Read the model definition and answer for the solid it produces. Units are mm, in the model's axes. Face numbers are marked on the shaded views. A direction names the side the tool comes from. Give positions to 0.01 mm unless a question says otherwise; leave off trailing zeros. Order: outer loops, then holes, each group sorted by start corner. A loop starts at its lowest first (then second) coordinate and runs counter-clockwise, first axis right, second up.
Item 1: A cutting plane is placed at D-D (x = 8). Write down the section's boundary in (y, z) (3 decimals), plus the area to 3 significant figures.
Item 2: A cutting plane is placed at C-C (x = 3.5). Write down the section's boundary in (y, z) (3 decimals).
Item 3: A cutting plane is placed at B-B (z = -2). Write down the section's boundary in (x, y) (3 decimals).
Item 4: Given pin 1 Ø2 at (x, z) = (7.5, -8) entering from +Y, flat-ended and moving along its own axis, determine where the tip first touches the part or whether it passes through.
Item 5: Find the intervals of material crossed by line 1 along X through (y, z) = (0.8, -1.5) (3 decimals); line 2 along Z through (x, y) = (6.5, 0.45) (3 decimals); line 3 along Z through (x, y) = (10.25, 0.7) (3 decimals), in increasing order.
Item 6: A cutting plane is placed at A-A (y = 1.1). Write down the section's boundary in (x, z) (3 decimals), plus the area to 3 significant figures.
Item 7: The mould has two halves that part along Z. Classify the marked faces 3, 4 and 5: +Z half, -Z half, draft (parallel to the pull), parting line (faces both ways), or undercut.
Item 8: Which of the six approach directions +Z, -Z, +X, -X, +Y, -Y give full straight-line access (tool end or side, diameter ignored) to the marked faces 1 and 2?
from build123d import *

# Parameters (mm, degrees)
SKETCH1_W           = 12.7
SKETCH1_H           = 12.7
BOSS_EXTRUDE1_DEPTH = 2.54
FILLET1_R           = 0.635
SHELL1_START        = 0.635
SHELL1_OUTLINE_W    = 1.905
SHELL1_OUTLINE_H    = 11.43
SHELL1_DEPTH        = 11.43
SKETCH2_R           = 2.54
BOSS_EXTRUDE2_DEPTH = 1.905
BOSS_EXTRUDE3_DEPTH = 0.00254


# Read off the part's stored shape, not the designer's step: Shell1
with BuildPart() as part:
    # Sketch1 → Boss-Extrude1 (new body)
    with BuildSketch(Plane(origin=(0, 0, 0), x_dir=(1, 0, 0), z_dir=(0, 1, 0))):
        with Locations((6.35, 6.35)):
            Rectangle(SKETCH1_W, SKETCH1_H)
    extrude(amount=BOSS_EXTRUDE1_DEPTH)

    # Fillet1
    fillet1_edges = [part.edges().sort_by_distance(p)[0] for p in [
        (0, 1.27, -12.7),
        (12.7, 1.27, -12.7),
        (12.7, 1.27, 0),
        (0, 1.27, 0),
    ]]
    fillet(fillet1_edges, radius=FILLET1_R)

    # Shell1 outline → Shell1 (cut)
    with BuildSketch(Plane.YZ.offset(SHELL1_START)):
        with Locations((0.9525, -6.35)):
            Rectangle(SHELL1_OUTLINE_W, SHELL1_OUTLINE_H)
    extrude(amount=SHELL1_DEPTH, mode=Mode.SUBTRACT)

    # Sketch2 → Boss-Extrude2 (add)
    with BuildSketch(Plane(origin=(0, 1.905, 0), x_dir=(-1, 0, 0), z_dir=(0, -1, 0))):
        with Locations(Location((-6.35, 6.35, 0), (0, 0, 270))):
            Circle(SKETCH2_R)
    extrude(amount=BOSS_EXTRUDE2_DEPTH)

    # Sketch3 → Boss-Extrude3 (add)
    with BuildSketch(Plane(origin=(0, 2.54, 0), x_dir=(1, 0, 0), z_dir=(0, 1, 0))):
        with BuildLine():
            Line((6.947551282, 7.576776242), (6.521419471, 7.186897436))
            add(Edge.make_bspline(
                [(6.521419471, 7.186897436), (6.503165812, 7.21264612), (6.468121331, 7.262080004), (6.411317883, 7.328273139), (6.354770931, 7.384740809), (6.297956603, 7.431247119), (6.240371318, 7.467509507), (6.182115036, 7.493183679), (6.123518028, 7.509504993), (6.084149883, 7.51153739), (6.064758814, 7.512538462)],
                knots=[0, 0, 0, 0, 1.299362458, 2.494594718, 3.587462134, 4.587049575, 5.512617175, 6.380583204, 7.202344345, 8, 8, 8, 8], degree=3))
            add(Edge.make_bspline(
                [(6.064758814, 7.512538462), (6.046671381, 7.511904137), (6.0117493, 7.510679422), (5.961965283, 7.498505847), (5.917766323, 7.477496044), (5.879195557, 7.45002396), (5.84864182, 7.416926467), (5.82424703, 7.382215707), (5.810510714, 7.343902879), (5.808702744, 7.317588082), (5.807807692, 7.304560697)],
                knots=[0, 0, 0, 0, 1.185010067, 2.2879431, 3.333075148, 4.379039566, 5.372662701, 6.27520591, 7.14612461, 8, 8, 8, 8], degree=3))
            add(Edge.make_bspline(
                [(5.807807692, 7.304560697), (5.808368576, 7.291345451), (5.809498118, 7.264731783), (5.820407957, 7.225726137), (5.836852199, 7.18761308), (5.852565344, 7.164411849), (5.860597155, 7.152552484)],
                knots=[0, 0, 0, 0, 0.967525499, 1.948461899, 2.951351359, 4, 4, 4, 4], degree=3))
            add(Edge.make_bspline(
                [(5.860597155, 7.152552484), (5.867898941, 7.143334324), (5.884706688, 7.122115336), (5.916755618, 7.088507766), (5.957002343, 7.047335552), (6.006995642, 7.000014485), (6.064660156, 6.944842714), (6.132668709, 6.883989063), (6.209063719, 6.815568965), (6.263363522, 6.767923686), (6.291817107, 6.742957131)],
                knots=[0, 0, 0, 0, 0.473873513, 1.090794244, 1.870441696, 2.795289791, 3.865433203, 5.087734844, 6.473946851, 8, 8, 8, 8], degree=3))
            add(Edge.make_bspline(
                [(6.291817107, 6.742957131), (6.31852489, 6.719842892), (6.369210714, 6.675976869), (6.441326575, 6.613716092), (6.504704406, 6.557701589), (6.560267478, 6.508774018), (6.607173508, 6.466420016), (6.645619689, 6.430437133), (6.676075577, 6.401525888), (6.693387966, 6.384063478), (6.700776442, 6.376610978)],
                knots=[0, 0, 0, 0, 1.543621617, 2.929473131, 4.163658386, 5.240097082, 6.164993805, 6.925417477, 7.541396219, 8, 8, 8, 8], degree=3))
            add(Edge.make_bspline(
                [(6.700776442, 6.376610978), (6.72880678, 6.346276149), (6.782690932, 6.287961956), (6.852721334, 6.197593297), (6.910358621, 6.109375058), (6.954947919, 6.021647272), (6.98862355, 5.9331442), (7.012365316, 5.84169531), (7.026584417, 5.746345018), (7.02816307, 5.681280084), (7.028961538, 5.648370793)],
                knots=[0, 0, 0, 0, 1.206664779, 2.319633467, 3.337109185, 4.282041471, 5.190008762, 6.099243693, 7.03861361, 8, 8, 8, 8], degree=3))
            add(Edge.make_bspline(
                [(7.028961538, 5.648370793), (7.028393209, 5.616304725), (7.027278125, 5.553389906), (7.013620483, 5.46132344), (6.994145488, 5.373211837), (6.96403373, 5.290013874), (6.927333696, 5.210363884), (6.881324904, 5.135502559), (6.827293886, 5.064672272), (6.765366044, 4.999139201), (6.696866497, 4.939672482), (6.623394222, 4.886733804), (6.544230772, 4.843026182), (6.460052505, 4.807036073), (6.370904481, 4.77931601), (6.276892901, 4.7588283), (6.17787397, 4.746531899), (6.110163397, 4.745246456), (6.075571114, 4.744589744)],
                knots=[0, 0, 0, 0, 1.043214005, 2.046824704, 3.02475056, 3.976699089, 4.921714032, 5.875962561, 6.831408892, 7.817874052, 8.806269674, 9.781291748, 10.760897367, 11.74438705, 12.757449933, 13.795994037, 14.874007457, 16, 16, 16, 16], degree=3))
            add(Edge.make_bspline(
                [(6.075571114, 4.744589744), (6.048416466, 4.745071485), (5.994634689, 4.74602561), (5.915368481, 4.753815242), (5.838827997, 4.766386881), (5.765099453, 4.784405794), (5.693850688, 4.807238201), (5.625078777, 4.835127112), (5.559258474, 4.868504794), (5.495891752, 4.906684869), (5.435286652, 4.951016965), (5.376676846, 5.000594728), (5.320644503, 5.056180684), (5.266920509, 5.117643377), (5.215848607, 5.185156853), (5.165757029, 5.257780861), (5.118871997, 5.336863206), (5.089909027, 5.392340111), (5.075115385, 5.420676482)],
                knots=[0, 0, 0, 0, 1.016823716, 2.013894106, 2.979844003, 3.91962641, 4.853723003, 5.779685073, 6.695824784, 7.614987388, 8.547259901, 9.504950863, 10.487499108, 11.500346958, 12.559593716, 13.656357062, 14.802919212, 16, 16, 16, 16], degree=3))
            Line((5.075115385, 5.420676482), (5.576297276, 5.721512821))
            add(Edge.make_bspline(
                [(5.576297276, 5.721512821), (5.594801911, 5.689347337), (5.630276879, 5.627683355), (5.690392527, 5.54482998), (5.751977941, 5.473879779), (5.816456918, 5.416086802), (5.883045419, 5.370678281), (5.952065082, 5.338226202), (6.023564398, 5.318138402), (6.072266484, 5.315685218), (6.096559696, 5.314461538)],
                knots=[0, 0, 0, 0, 1.283663364, 2.460892379, 3.537111102, 4.529833553, 5.449777664, 6.316464042, 7.160231139, 8, 8, 8, 8], degree=3))
            add(Edge.make_bspline(
                [(6.096559696, 5.314461538), (6.12126937, 5.315460861), (6.169209736, 5.317399693), (6.237638475, 5.335308096), (6.300376534, 5.363425604), (6.354606849, 5.403545409), (6.40052566, 5.449849762), (6.434416378, 5.501365473), (6.455706756, 5.557104227), (6.457957665, 5.595824033), (6.459089744, 5.615297877)],
                knots=[0, 0, 0, 0, 1.13588714, 2.203786484, 3.234766741, 4.283437687, 5.291419208, 6.222934724, 7.106237994, 8, 8, 8, 8], degree=3))
            add(Edge.make_bspline(
                [(6.459089744, 5.615297877), (6.458044316, 5.633415119), (6.455920629, 5.670218563), (6.440278206, 5.724939365), (6.415824328, 5.779635282), (6.386893665, 5.824498352), (6.357453094, 5.862060985), (6.329301267, 5.894607307), (6.295019789, 5.930565296), (6.254695583, 5.969980182), (6.208861436, 6.013198947), (6.157478739, 6.060217356), (6.099959106, 6.110621236), (6.059304117, 6.14495586), (6.038046074, 6.162909054)],
                knots=[0, 0, 0, 0, 0.916159276, 1.861089862, 2.860218735, 3.940849679, 4.552606315, 5.27541173, 6.11797699, 7.06649574, 8.129236253, 9.306560635, 10.591630461, 12, 12, 12, 12], degree=3))
            add(Edge.make_bspline(
                [(6.038046074, 6.162909054), (5.997633688, 6.197101808), (5.920070088, 6.262728051), (5.810462881, 6.359655946), (5.711696974, 6.450243946), (5.624625414, 6.535611915), (5.548138776, 6.614183306), (5.482755059, 6.686596305), (5.429192535, 6.75340948), (5.372829528, 6.832545214), (5.319273403, 6.928977544), (5.272985712, 7.044996816), (5.242956212, 7.161001367), (5.239591824, 7.238880433), (5.237935897, 7.277211939)],
                knots=[0, 0, 0, 0, 1.345494975, 2.582412109, 3.71882943, 4.751509156, 5.681369928, 6.505683931, 7.230279997, 7.856715994, 8.973648664, 10.023341002, 11.027102913, 12, 12, 12, 12], degree=3))
            add(Edge.make_bspline(
                [(5.237935897, 7.277211939), (5.238624595, 7.304394586), (5.239981404, 7.35794732), (5.252084347, 7.436688812), (5.270172657, 7.512667736), (5.296442076, 7.585606886), (5.33053661, 7.655414903), (5.371943098, 7.722433526), (5.421304502, 7.786045931), (5.476931473, 7.846209948), (5.538218153, 7.901193012), (5.603710758, 7.949721076), (5.673038596, 7.990708584), (5.745777553, 8.024710699), (5.822378363, 8.050737157), (5.90227671, 8.069186008), (5.985587195, 8.080158796), (6.042253188, 8.08165042), (6.07111899, 8.082410256)],
                knots=[0, 0, 0, 0, 1.010766082, 1.991317756, 2.957454644, 3.913069143, 4.869106762, 5.843196583, 6.838735724, 7.860187025, 8.887984031, 9.89767229, 10.887916223, 11.879572884, 12.879850636, 13.892031539, 14.926195476, 16, 16, 16, 16], degree=3))
            add(Edge.make_bspline(
                [(6.07111899, 8.082410256), (6.108527641, 8.081041768), (6.183049652, 8.078315594), (6.293232593, 8.056997805), (6.400854684, 8.023473336), (6.487578582, 7.983029753), (6.556583169, 7.943852034), (6.609468739, 7.907782126), (6.663282653, 7.866462108), (6.718458887, 7.819761769), (6.773972181, 7.766801214), (6.831401043, 7.70884121), (6.889962936, 7.645380848), (6.92801888, 7.600045059), (6.947551282, 7.576776242)],
                knots=[0, 0, 0, 0, 1.282922637, 2.555718331, 3.837320111, 5.142675274, 5.830281639, 6.55870424, 7.337177975, 8.157850921, 9.037902056, 9.96903443, 10.957596896, 12, 12, 12, 12], degree=3))
        make_face()
    extrude(amount=BOSS_EXTRUDE3_DEPTH)


solid = part.part
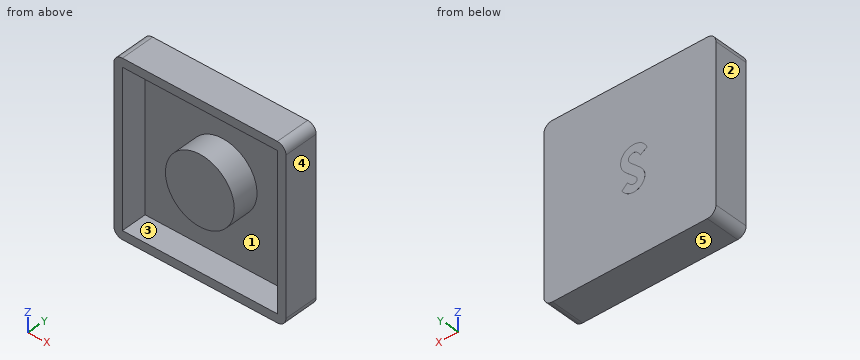
Response values:
1. outline: (0, -12.7) - (2.54, -12.7) - (2.54, 0) - (0, 0) - (0, -0.635) - (1.905, -0.635) - (1.905, -4.419) - (0, -4.419) - (0, -8.281) - (1.905, -8.281) - (1.905, -12.065) - (0, -12.065) - close
1. area: 17.8 mm2
2. outline: (0, -12.7) - (2.54, -12.7) - (2.54, 0) - (0, 0) - (0, -0.635) - (1.905, -0.635) - (1.905, -12.065) - (0, -12.065) - close
3. outline: (0, 0) - (0.635, 0) - (0.635, 1.905) - (12.065, 1.905) - (12.065, 0) - (12.7, 0) - (12.7, 2.54) - (0, 2.54) - close
4. pin 1: stops at y = 2.54
5. line 1: x = 0 to 0.635, 12.065 to 12.7
5. line 2: z = -12.7 to -12.065, -8.886 to -3.814, -0.635 to 0
5. line 3: z = -12.7 to -12.065, -0.635 to 0
6. outline: (0, -12.065) arc R0.635 ccw to (0.635, -12.7) - (12.065, -12.7) arc R0.635 ccw to (12.7, -12.065) - (12.7, -0.635) arc R0.635 ccw to (12.065, 0) - (0.635, 0) arc R0.635 ccw to (0, -0.635) - close; circle Ø5.08 at (6.35, -6.35); hole (0.635, -12.065) - (12.065, -12.065) - (12.065, -0.635) - (0.635, -0.635) - close
6. area: 50.6 mm2
7. face 3: undercut
7. face 4: draft
7. face 5: -Z half
8. face 1: -Y
8. face 2: +Z, -Z, -X, +Y, -Y
